Source: CAD feature listing. Evaluate the final solid. Frame: model axes, mm. A direction names the side the tool comes from. Round coordinates to 2 decimals unless told otherwise and drop trailing zeros. Order: outer loops, then holes, each group sorted by start corner. A loop starts at its lowest first (then second) coordinate and runs counter-clockwise, first axis right, second up. Notation, with made-up numbers: (74.25, -14.75) -> (115.25, -14.75) arc R13 ccw to (115.25, 1.25) -> close; hole circle Ø2 at (80.25, -5.75). An arc over 180 degrees is marked (long way). Write item = value, one per line. Start each with the question number.
(1) Draft query along Y for faces 3 (the face through (-2, -50.8, -6)), 4 (the face through (-2, -22, 0)), 5 (the face through (-11.092, -8.505, -6.261)). Return one class per face: released by +Y, released by -Y, zero draft, split by the parting line, or undercut.
(2) Cut plane B-B on x = -57.15. Return the cut outline in (y, z) (3 decimals).
(3) Contact query for a flat-ended pin moving along its axis: pin 1 Ø2 at (x, y) = (-20.5, -6.5) entering from +Z. Output: stop coordinate, or through.
(4) Reachability of faces 1 (the face through (-2, -22, -12.7)), 2 (the face through (86.48, -12.16, -1.57)) from +Z, -Z, +X, -X, +Y, -Y: full face, straight path, thin tool, end or side. Return the list, or none.
(5) Cut plane C-C on x = 74. Return the cut outline in (y, z) (3 decimals).
(6) Cut plane A-A on z = -5.5. Return the cut outline in (x, y) (3 decimals), then the cut area to 3 significant figures.
(7) Ray query, line 1 (Y direction, x = -114.3, z = -3); line 2 (Y direction, x = 57.15, z = -0.7); line 3 (Y direction, x = 57.15, z = -10.5) (3 decimals). Return the intervals inside material, ascending.
from build123d import *

# Parameters (mm, degrees)
SKETCH4_W          = 254
SKETCH4_H          = 101.6
BASE_EXTRUDE_DEPTH = 12.7
SKETCH5_R          = 28.575
SKETCH5_R_2        = 13.977315316
CUT_EXTRUDE1_DEPTH = 12.7
SKETCH6_R          = 31.75
CUT_EXTRUDE2_DEPTH = 3.175
SKETCH7_R          = 2.0193
CUT_EXTRUDE3_DEPTH = 25.4


with BuildPart() as part:
    # Sketch4 → Base-Extrude (new body)
    with BuildSketch(Plane.XY):
        Rectangle(SKETCH4_W, SKETCH4_H)
    extrude(amount=-BASE_EXTRUDE_DEPTH)

    # Sketch5 → Cut-Extrude1 (cut)
    with BuildSketch(Plane.XY):
        with Locations((-57.15, 0)):
            Circle(SKETCH5_R)
        with Locations((57.15, 0)):
            Circle(SKETCH5_R)
        Circle(SKETCH5_R_2)
    extrude(amount=-CUT_EXTRUDE1_DEPTH, mode=Mode.SUBTRACT)

    # Sketch6 → Cut-Extrude2 (cut)
    with BuildSketch(Plane.XY):
        with Locations((-57.15, 0)):
            Circle(SKETCH6_R)
        with Locations((57.15, 0)):
            Circle(SKETCH6_R)
    extrude(amount=-CUT_EXTRUDE2_DEPTH, mode=Mode.SUBTRACT)

    # Sketch7 → Cut-Extrude3 (cut)
    with BuildSketch(Plane.XY):
        with Locations((-114.3, -38.1)):
            Circle(SKETCH7_R)
        with Locations((-114.3, 38.1)):
            Circle(SKETCH7_R)
        with Locations((114.3, -38.1)):
            Circle(SKETCH7_R)
        with Locations((114.3, 38.1)):
            Circle(SKETCH7_R)
    extrude(amount=-CUT_EXTRUDE3_DEPTH, mode=Mode.SUBTRACT)


solid = part.part
Evaluation:
q1.face_3 = released by -Y
q1.face_4 = zero draft
q1.face_5 = undercut
q2.outline = (-50.8, -12.7) -> (-28.575, -12.7) -> (-28.575, -3.175) -> (-31.75, -3.175) -> (-31.75, 0) -> (-50.8, 0) -> close; (28.575, -12.7) -> (50.8, -12.7) -> (50.8, 0) -> (31.75, 0) -> (31.75, -3.175) -> (28.575, -3.175) -> close
q3.pin_1 = 0
q4.face_1 = -Z, +X, -X, +Y, -Y
q4.face_2 = +Z
q5.outline = (-50.8, -12.7) -> (-23.078, -12.7) -> (-23.078, -3.175) -> (-26.91, -3.175) -> (-26.91, 0) -> (-50.8, 0) -> close; (23.078, -12.7) -> (50.8, -12.7) -> (50.8, 0) -> (26.91, 0) -> (26.91, -3.175) -> (23.078, -3.175) -> close
q6.outline = (-127, -50.8) -> (127, -50.8) -> (127, 50.8) -> (-127, 50.8) -> close; hole circle Ø4.039 at (-114.3, -38.1); hole circle Ø4.039 at (-114.3, 38.1); hole circle Ø57.15 at (-57.15, 0); hole circle Ø27.955 at (0, 0); hole circle Ø57.15 at (57.15, 0); hole circle Ø4.039 at (114.3, -38.1); hole circle Ø4.039 at (114.3, 38.1)
q6.area = 20,000 mm^2
q7.line_1 = -50.8 to -40.12, -36.08 to 36.08, 40.12 to 50.8
q7.line_2 = -50.8 to -31.75, 31.75 to 50.8
q7.line_3 = -50.8 to -28.575, 28.575 to 50.8
